The listing builds one solid part. Answer for the finished solid, in the listing's coordinates (mm). Round coordinates to 2 decimals unless told otherwise and drop trailing zeros. Loops run counter-clockwise (first coordinate to the right, second up) from the corner with the lowest first, then second, coordinate; pieces in that order, holes last. Notation, with made-up numbers: (-11.5, -39.75) - (30.5, -39.75) arc R22 ccw to (30.5, -33.75) - close; hole circle Ø7 at (75.25, 10.25). An arc over 180 degrees is marked (long way). One line per question, with ' | ' between items. Start each with the question number.
Autodesk Inventor part; units mm, degrees
ref_plane "YZ Plane" through (0, 0, 0) normal (1, 0, 0) x (0, 1, 0)
ref_plane "XZ Plane" through (0, 0, 0) normal (0, 1, 0) x (-1, 0, 0)
ref_plane "XY Plane" through (0, 0, 0) normal (0, 0, 1) x (1, 0, 0)
sketch "Sketch1" plane through (0, 0, 0) normal (0, 0, 1) x (1, 0, 0)
  circle A0 centre (0, 0) radius 1.905
  line L0 (0, 0) -> (6.35, 0)
  line L1 (6.35, 0) -> (-6.35, 0)
  circle A1 centre (-6.35, 0) radius 1.5875
  circle A2 centre (6.35, 0) radius 1.5875
  line L2 (-9.525, 3.175) -> (9.525, 3.175)
  line L3 (9.525, 3.175) -> (9.525, -3.175)
  line L4 (9.525, -3.175) -> (-9.525, -3.175)
  line L5 (-9.525, -3.175) -> (-9.525, 3.175)
  dimension "d0" = 3.81
  dimension "d1" = 6.35
  dimension "d2" = 12.7
  dimension "d3" = 3.175
  dimension "d4" = 3.175
  dimension "d5" = 19.05
  dimension "d6" = 9.525
  dimension "d7" = 6.35
  dimension "d8" = 3.175
sketch "Sketch1 outline for Extrusion1" plane through (0, 0, 0) normal (0, 0, 1) x (1, 0, 0)
  line L0 (-9.525, 3.175) -> (9.525, 3.175)
  line L1 (-9.525, -3.175) -> (-9.525, 3.175)
  line L2 (9.525, 3.175) -> (9.525, -3.175)
  line L3 (9.525, -3.175) -> (-9.525, -3.175)
  circle A0 centre (-6.35, 0) radius 1.5875
  circle A1 centre (0, 0) radius 1.905
  circle A2 centre (6.35, 0) radius 1.5875
extrude "Extrusion1" add sketch "Sketch1 outline for Extrusion1" along normal blind 1.5875
chamfer "Chamfer1" distance 1.27 angle 45 2 edges at (-7.9375, 0, 1.5875) (4.7625, 0, 1.5875)
fillet "Fillet1" radius 3.175 4 edges at (-9.525, 3.175, 0.7937) (-9.525, -3.175, 0.7937) (9.525, -3.175, 0.7937) (9.525, 3.175, 0.7937)
properties part number "pushSwitchBushingHolderRear" material "ABS Plastic"
(1) Find section A-A on x = 0. Write down the section's boundary in (y, z) (1 decimal).
(2) Determine the mould class of faces 1 (the cylindrical face through (8.62, 2.22, 0.8)), 2 (the cylindrical face through (-0.41, 1.86, 0.78)), 3 (the cylindrical face through (-4.836, -0.477, 0.157)), 4 (the cylindrical face through (-8.62, -2.22, 0.8)) for opening direction Y: pulls with the +Y half, pulls with the -Y half, needs draft (parallel to the pull), parting line crosses it, or undercut.
(3) Find section B-B on z = 0.8. Count the separate pieces of the cut face and the enclosed holes in it, plus the area to 3 significant figures.
(4) Consider L1, parallel to Y at x = -6.35, z = 0.25 (1 decimal); L2, parallel to X at y = -1, z = 0.4; L3, parallel to X at y = -1.5, z = 1.3. Determine where each line is inside the solid, lowest interval first.
Answer below:
1) outline: (-3.2, 0) - (-1.9, 0) - (-1.9, 1.6) - (-3.2, 1.6) - close; (1.9, 0) - (3.2, 0) - (3.2, 1.6) - (1.9, 1.6) - close
2) face 1: pulls with the +Y half | face 2: undercut | face 3: undercut | face 4: pulls with the -Y half
3) separate pieces: 1 | enclosed holes: 3 | area: 74.0 mm2
4) L1: -3.2 to -1.6, 1.6 to 3.2 | L2: -9.36 to -7.69, -5.01 to -1.62, 1.62 to 5.01, 7.69 to 9.36 | L3: -9.15 to -8.44, -4.26 to -1.17, 1.17 to 4.26, 8.44 to 9.15
